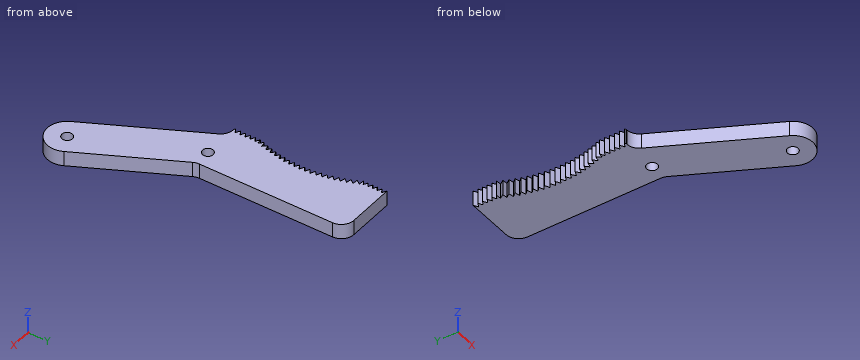
```python
from build123d import *

# Parameters (mm, degrees)
SKETCH1_R           = 2.15
BOSS_EXTRUDE1_DEPTH = 6
CUT_EXTRUDE1_DEPTH  = 65.899922958
LPATTERN1_COUNT     = 5
LPATTERN1_PITCH     = 1.85
FILLET1_R           = 5
CUT_EXTRUDE2_DEPTH  = 65.899922958
CIRPATTERN1_COUNT   = 20
CIRPATTERN1_ANGLE   = 47
CUT_EXTRUDE3_DEPTH  = 65.899922958
LPATTERN2_COUNT     = 8
LPATTERN2_PITCH     = 2


with BuildPart() as part:
    # Sketch1 → Boss-Extrude1 (new body)
    with BuildSketch(Plane.XY):
        with BuildLine():
            Line((0, 60), (0, 0))
            Line((0, 0), (20.330487993, -39.021420502))
            ThreePointArc((20.330487993, -39.021420502), (16.932136627, -49.812676592), (6.140880537, -46.414325226))
            Line((6.140880537, -46.414325226), (-18.041372942, 0))
            Line((-18.041372942, 0), (-22.041372942, 0))
            Line((-22.041372942, 0), (-22.041372942, 11.19846791))
            ThreePointArc((-22.041372942, 11.19846791), (-18.769082447, 31.167731967), (-24, 50.715542423))
            Line((-24, 50.715542423), (-24, 60))
            Line((-24, 60), (0, 60))
        make_face()
        with Locations((-6.63687696, 0)):
            Circle(SKETCH1_R, mode=Mode.SUBTRACT)
        with Locations((13.235684265, -42.717872864)):
            Circle(SKETCH1_R, mode=Mode.SUBTRACT)
    extrude(amount=BOSS_EXTRUDE1_DEPTH)

    # Sketch2 → Cut-Extrude1 (cut, through all)
    with BuildSketch(Plane.XY.offset(6)):
        Polygon((-24, 60), (-22.267949192, 59), (-24, 58), align=None)
    cut_extrude1 = extrude(amount=-CUT_EXTRUDE1_DEPTH, mode=Mode.SUBTRACT)

    # LPattern1: Cut-Extrude1 ×5
    with Locations(*[(0, -i * LPATTERN1_PITCH, 0) for i in range(1, LPATTERN1_COUNT)]):
        add(cut_extrude1, mode=Mode.SUBTRACT)

    # Fillet1
    fillet1_edges = [part.edges().sort_by_distance(p)[0] for p in [
        (0, 60, 3),
        (0, 0, 3),
        (-18.041372942, 0, 3),
    ]]
    fillet(fillet1_edges, radius=FILLET1_R)

    # Sketch3 → Cut-Extrude2 (cut, through all)
    with BuildSketch(Plane.XY.offset(6)):
        Polygon((-23.954411467, 50.626320552), (-21.741449412, 50.459283267), (-22.992588972, 48.626320552), align=None)
    cut_extrude2 = extrude(amount=-CUT_EXTRUDE2_DEPTH, mode=Mode.SUBTRACT)

    # CirPattern1: Cut-Extrude2 ×20 about axis
    cirpattern1_axis = Axis((-66.806944036, 28.78678002, 0), (0, 0, -1))
    for i in range(1, CIRPATTERN1_COUNT):
        add(cut_extrude2.rotate(cirpattern1_axis, i * CIRPATTERN1_ANGLE / (CIRPATTERN1_COUNT - 1)), mode=Mode.SUBTRACT)

    # Sketch4 → Cut-Extrude3 (cut, through all)
    with BuildSketch(Plane.XY.offset(6)):
        Polygon((-22.041372942, 10.33072384), (-20.309322134, 9.33072384), (-22.041372942, 8.33072384), align=None)
    cut_extrude3 = extrude(amount=-CUT_EXTRUDE3_DEPTH, mode=Mode.SUBTRACT)

    # LPattern2: Cut-Extrude3 ×8
    with Locations(*[(0, -i * LPATTERN2_PITCH, 0) for i in range(1, LPATTERN2_COUNT)]):
        add(cut_extrude3, mode=Mode.SUBTRACT)


solid = part.part
```
Source: CAD feature listing. Evaluate the final solid. Frame: model axes, mm. Give positions to 0.01 mm unless a question says otherwise; leave off trailing zeros. Write each loop counter-clockwise with the first axis right and the second up, starting at its lowest first coordinate (ties: lowest second). Pieces come first, ordered by that corner, then holes.
1. Material intervals for line 1 along Y through (x, z) = (-20, 2.75); line 2 along Y through (x, z) = (-9, 2.75); line 3 along X through (y, z) = (4.5, 4), sorted ascending.
2. Section query B-B (z = 3.5). Count the separate pieces of the cut face and the enclosed holes in it, then the cut area to 3 significant figures.
3. Section query C-C (y = -34). Return the cut outline in (x, z).
4. First-contact query: pin 1 (4 mm diameter, centred on x = -5, y = -11.5, fed in from -Z); pin 2 (4 mm diameter, centred on x = -6.64, y = 0, fed in from -Z); pin 3 (1 mm diameter, centred on x = 1.5, z = 4, fed in from -Y); pin 4 (3 mm diameter, centred on y = 28.5, z = 2, fed in from +X). Flat tips, straight axial feed; report the tip coordinate or a pass-through.
5. Section query A-A (x = -10). Return the cut outline in (y, z), then the cut area to 3 significant figures.
Output values:
1. line 1: y = -0.12 to 12.53, 13.23 to 14.41, 15.92 to 16.28, 40.86 to 41.04, 42.73 to 43.69, 44.6 to 60
1. line 2: y = -17.35 to 60
1. line 3: x = -21.75 to 0
2. separate pieces: 1
2. enclosed holes: 2
2. area: 2,050 mm2
3. outline: (-0.33, 0) - (17.71, 0) - (17.71, 6) - (-0.33, 6) - close
4. pin 1: stops at z = 0
4. pin 2: passes through
4. pin 3: stops at y = -38.47
4. pin 4: stops at x = 0
5. outline: (-15.43, 0) - (60, 0) - (60, 6) - (-15.43, 6) - close
5. area: 453 mm2
